Source: three-view drawing plus pictorial views. Frame: mm from the lowest corner of the part. Coordinates: 2 decimals unless noted, no trailing zeros. Loops run counter-clockwise (first coordinate to the right, second up) from the corner with the lowest first, then second, coordinate; pieces in that order, holes last. Notation, with made-up numbers: (40, 52.5) - (88, 52.5) arc R15 cw to (88, 71.5) - close; hole circle Ø1 at (8.5, 61). An arc over 180 degrees is marked (long way). Return JSON: item names as keys, results as strings.
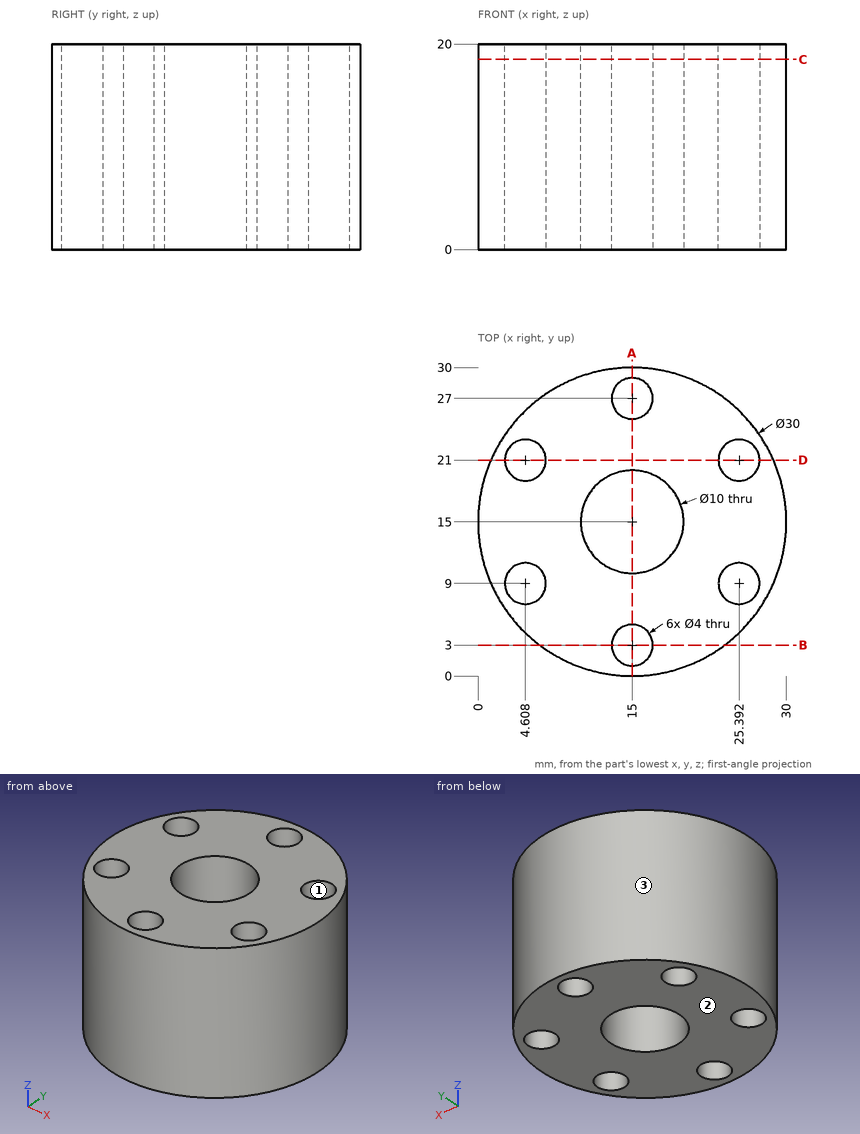
Item 1: Section query A-A, the plane x = 15. Return loops of the section in (y, z).
Worked out:
{"outline": "(0, 0) - (1, 0) - (1, 20) - (0, 20) - close; (5, 0) - (10, 0) - (10, 20) - (5, 20) - close; (20, 0) - (25, 0) - (25, 20) - (20, 20) - close; (29, 0) - (30, 0) - (30, 20) - (29, 20) - close"}
Item 2: Section query B-B, the plane y = 3. Return loops of the section in (x, z).
Worked out:
{"outline": "(6, 0) - (13, 0) - (13, 20) - (6, 20) - close; (17, 0) - (24, 0) - (24, 20) - (17, 20) - close"}
Item 3: Mould query, pull axis X, two halves, no side actions, for the marked faces 1, 2 and 3. Classes: +X half, -X half, draft (parallel to the pull), parting line (faces both ways), or undercut.
Worked out:
{"face 1": "undercut", "face 2": "draft", "face 3": "parting line"}
Item 4: Section query D-D, the plane y = 21. Return loops of the section in (x, z).
Worked out:
{"outline": "(1.25, 0) - (2.61, 0) - (2.61, 20) - (1.25, 20) - close; (6.61, 0) - (23.39, 0) - (23.39, 20) - (6.61, 20) - close; (27.39, 0) - (28.75, 0) - (28.75, 20) - (27.39, 20) - close"}
Item 5: Section query C-C, the plane z = 18.5. Return loops of the section in (x, y).
Worked out:
{"outline": "circle Ø30 at (15, 15); hole circle Ø4 at (4.61, 9); hole circle Ø4 at (4.61, 21); hole circle Ø10 at (15, 15); hole circle Ø4 at (15, 3); hole circle Ø4 at (15, 27); hole circle Ø4 at (25.39, 9); hole circle Ø4 at (25.39, 21)"}
Item 6: First-contact query: pin 1 Ø10 at (x, z) = (18.5, 15.5) entering from -Y; pin 2 Ø3 at (x, z) = (19.5, 5.5) entering from -Y; pin 3 Ø2 at (y, z) = (7, 13.5) entering from +X; pin 4 Ø4 at (x, z) = (26, 4.5) entering from -Y. Flat tips, straight axial feed; report the tip coordinate or a pass-through.
Worked out:
{"pin 1": "y = 0", "pin 2": "y = 0.3", "pin 3": "x = 28.27", "pin 4": "y = 3"}
Item 7: Ray query, probe 1 along Y at (x, z) = (15, 5); probe 2 along X at (y, z) = (20.5, 14.75) (1 decimal); probe 3 along X at (y, z) = (16.75, 10). Return the intervals inside material, ascending. Write a range as from..to.
Worked out:
{"probe 1": "0..1, 5..10, 20..25, 29..30", "probe 2": "1..2.7, 6.5..23.5, 27.3..29", "probe 3": "0.1..10.32, 19.68..29.9"}
